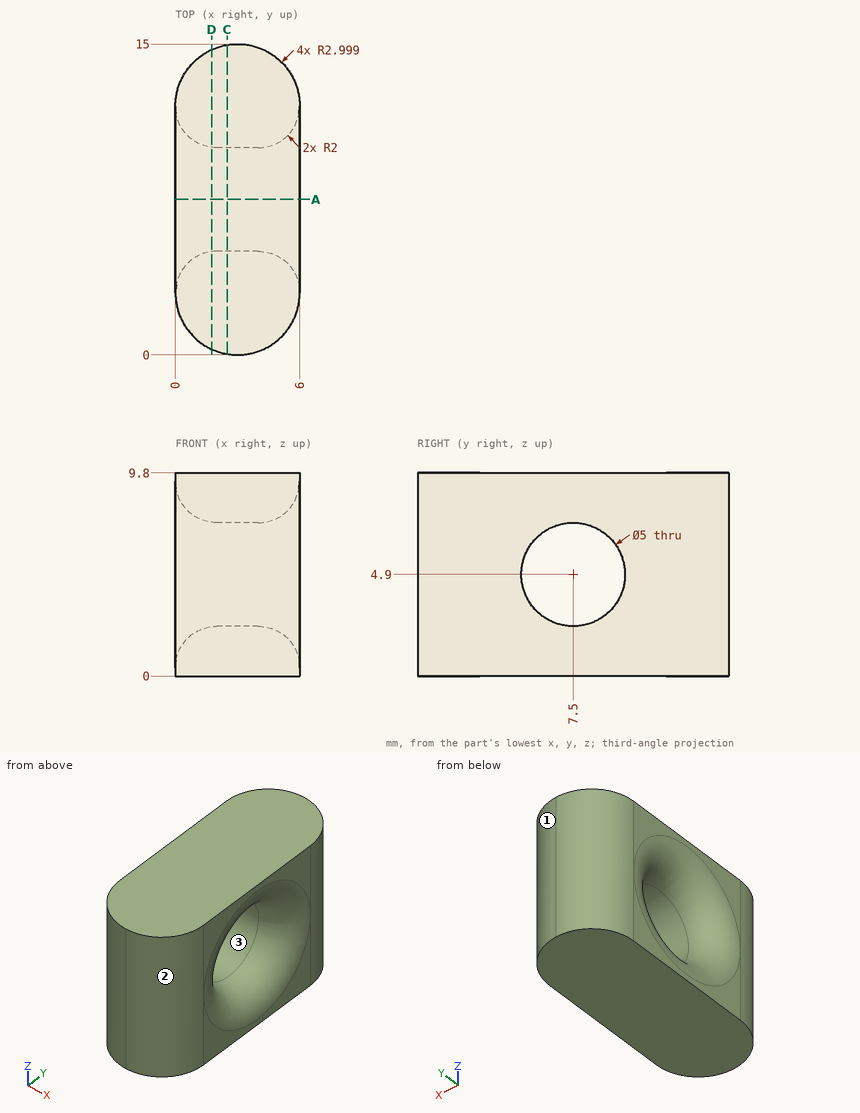
Check sheet for the drawn part. Datum: minimum x, y, z corner. Units: mm. Round coordinates to 2 decimals unless told otherwise and drop trailing zeros. Loops run counter-clockwise (first coordinate to the right, second up) from the corner with the lowest first, then second, coordinate; pieces in that order, holes last. Notation, with made-up numbers: M 60.5,59 L 106.5,59 A22 cw 106.5,75 Z; hole C 70,38 d9. An arc over 180 degrees is marked long. One line per question, with ' | ' between items. Start each with the question number.
Item 1: Section check A-A (y = 7.5). Record the boundary of the cut face in (x, z).
Item 2: Section check D-D (x = 1.75). Record the boundary of the cut face in (y, z) (1 decimal), and give its area (3 significant figures).
Item 3: Release check for a two-part mould opening along Y. For the marked faces 1, 2 and 3 record: released by +Y, released by -Y, zero draft, split by the parting line, or undercut.
Item 4: Scan lines: probe 1 along Z at (x, y) = (3, 7.5); probe 2 along Y at (x, z) = (3, 5); probe 3 along X at (y, z) = (7, 9.25). Record each from-to range of solid material in increasing order.
Item 5: Gauge pin test, flat end, axial feed: pin 1 Ø3 at (y, z) = (5.5, 6) entering from +X. Record the tip position at first contact, or that the pin passes through.
Item 6: Section check C-C (x = 2.5). Record the boundary of the cut face in (y, z).
Worked out:
1) outline: M 0,0 L 6,0 L 6,0.4 A2 ccw 4,2.4 L 2,2.4 A2 ccw 0,0.4 Z; M 0,9.4 A2 ccw 2,7.4 L 4,7.4 A2 ccw 6,9.4 L 6,9.8 L 0,9.8 Z
2) outline: M 0.3,0 L 14.7,0 L 14.7,9.8 L 0.3,9.8 Z; hole C 7.5,4.9 d5 | area: 122 mm^2
3) face 1: released by +Y | face 2: released by -Y | face 3: undercut
4) probe 1: 0 to 2.4, 7.4 to 9.8 | probe 2: 0 to 5, 10 to 15 | probe 3: 0 to 6
5) pin 1: x = 5.87
6) outline: M 0.04,0 L 14.96,0 L 14.96,9.8 L 0.04,9.8 Z; hole C 7.5,4.9 d5
